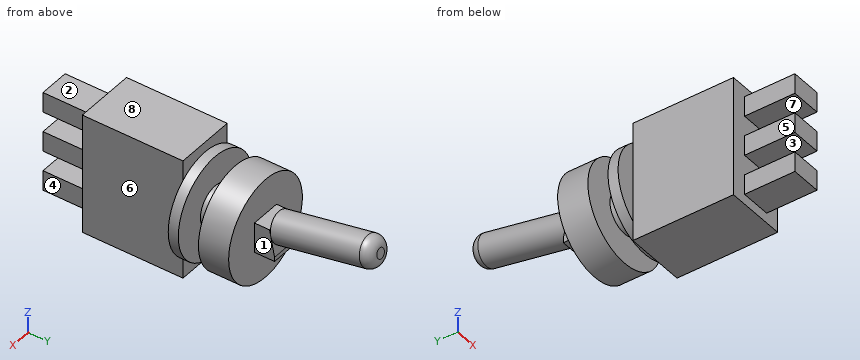
from build123d import *

# Parameters (mm, degrees)
ESQUISSE1_R      = 5
EXTRUSION1_DEPTH = 3
ESQUISSE3_R      = 2
EXTRUSION3_DEPTH = 2
ESQUISSE4_R      = 5
EXTRUSION4_DEPTH = 1
ESQUISSE5_W      = 6
ESQUISSE5_H      = 12
EXTRUSION5_DEPTH = 10
ESQUISSE6_W      = 3
ESQUISSE6_H      = 2
EXTRUSION6_DEPTH = 5
ESQUISSE8_W      = 3
ESQUISSE8_H      = 3
EXTRUSION8_DEPTH = 2
CHANFREIN1_SIZE  = 0.5
CHANFREIN1_SIZE2 = 2.572277008
ESQUISSE9_R      = 1.5
EXTRUSION9_DEPTH = 10
CONG_1_R         = 1


with BuildPart() as part:
    # Esquisse1 → Extrusion1 (new body)
    with BuildSketch(Plane(origin=(0, 0, 0), x_dir=(1, 0, 0), z_dir=(0, 1, 0))):
        Circle(ESQUISSE1_R)
    extrude(amount=EXTRUSION1_DEPTH)

    # Esquisse3 → Extrusion3 (add)
    with BuildSketch(Plane.XZ):
        Circle(ESQUISSE3_R)
    extrude(amount=EXTRUSION3_DEPTH)

    # Esquisse4 → Extrusion4 (add)
    with BuildSketch(Plane.XZ.offset(2)):
        Circle(ESQUISSE4_R)
    extrude(amount=EXTRUSION4_DEPTH)

    # Esquisse5 → Extrusion5 (add)
    with BuildSketch(Plane.XZ.offset(3)):
        Rectangle(ESQUISSE5_W, ESQUISSE5_H)
    extrude(amount=EXTRUSION5_DEPTH)

    # Esquisse6 → Extrusion6 (add)
    with BuildSketch(Plane.XZ.offset(13)):
        with Locations((0, 4)):
            Rectangle(ESQUISSE6_W, ESQUISSE6_H)
        Rectangle(ESQUISSE6_W, ESQUISSE6_H)
        with Locations((0, -4)):
            Rectangle(ESQUISSE6_W, ESQUISSE6_H)
    extrude(amount=EXTRUSION6_DEPTH)

    # Esquisse8 → Extrusion8 (add)
    with BuildSketch(Plane(origin=(0, 3, 0), x_dir=(-1, 0, 0), z_dir=(0, 1, 0))):
        Rectangle(ESQUISSE8_W, ESQUISSE8_H)
    extrude(amount=EXTRUSION8_DEPTH)

    # Chanfrein1
    chanfrein1_edges = [part.edges().sort_by_distance(p)[0] for p in [
        (0, 5, 1.5),
    ]]
    chanfrein1_side = [part.faces().sort_by_distance(p)[0] for p in [
        (0, 4, 1.5),
    ]]
    chamfer(chanfrein1_edges, length=CHANFREIN1_SIZE, length2=CHANFREIN1_SIZE2, reference=chanfrein1_side[0])

    # Esquisse9 → Extrusion9 (add)
    with BuildSketch(Plane(origin=(0, 4.617118618, 0.897476944), x_dir=(-1, 0, 0), z_dir=(0, 0.981627183, 0.190808995))):
        Circle(ESQUISSE9_R)
    extrude(amount=EXTRUSION9_DEPTH)

    # Congé1
    cong_1_edges = [part.edges().sort_by_distance(p)[0] for p in [
        (1.5, 14.433390452, 2.805566898),
    ]]
    fillet(cong_1_edges, radius=CONG_1_R)


solid = part.part
Part model, mm, in its own coordinate system. Face numbers are marked on the shaded views. A direction names the side the tool comes from. Give positions to 0.01 mm unless a question says otherwise; leave off trailing zeros. Loops run counter-clockwise (first coordinate to the right, second up) from the corner with the lowest first, then second, coordinate; pieces in that order, holes last. Notation, with made-up numbers: M 24.25,-16.5 L 34.25,-16.5 A28 ccw 34.25,9.5 Z; hole C 57,22 d10. An arc over 180 degrees is marked long. Put each result on its own line as item: value. Start each with the question number.
1) 3-axis set-ups, long thin cutter, end or side, ignore diameter. For the marked faces 1, 2, 3, 4 and 5: which of +Z, -Z, +X, -X, +Y, -Y reach the whole face in a straight line?
2) Pull direction Z, two halves, no side cores. Call the marked faces 6, 7 and 8: +Z half, -Z half, draft (parallel to the pull), parting line (faces both ways), or undercut.
3) Saw through at C-C (y = -8). List the corners of the cut face in (x, z), then the cut area to 3 significant figures.
4) Flat gauge pins, fed straight in: pin 1 (1.6 mm diameter, centred on x = -1.5, z = 5, fed in from +Y); pin 2 (0.8 mm diameter, centred on x = 0, y = 4, fed in from +Z); pin 3 (1.6 mm diameter, centred on y = -16, z = 4, fed in from -X). Where does each tip first touch, or does it go through?
5) Saw through at B-B (y = -1). List the corners of the cut face in (x, z), then the cut area to 3 significant figures.
6) Saw through at A-A (x = 4). List the corners of the cut face in (y, z).
7) Probe probe 1 along Z at (x, y) = (-0.5, -16); probe 2 along Y at (x, z) = (1.25, -4.5); probe 3 along Y at (x, z) = (2, -0.5). List the from-to ranges inside material, lowest first.
Numbers:
1. face 1: +Z, -Z, +X, +Y
1. face 2: +Z, +X, -X, -Y
1. face 3: +X, -X, -Y
1. face 4: +Z, -Z, +X, -Y
1. face 5: +Z, -Z, -X, -Y
2. face 6: draft
2. face 7: undercut
2. face 8: +Z half
3. outline: M -3,-6 L 3,-6 L 3,6 L -3,6 Z
3. area: 72.0 mm^2
4. pin 1: y = 3
4. pin 2: z = 2.38
4. pin 3: x = -1.5
5. outline: C 0,0 d4
5. area: 12.6 mm^2
6. outline: M -3,-3 L -2,-3 L -2,3 L -3,3 Z; M 0,-3 L 3,-3 L 3,3 L 0,3 Z
7. probe 1: -5 to -3, -1 to 1, 3 to 5
7. probe 2: -18 to -2, 0 to 3
7. probe 3: -13 to -2, 0 to 3
